```python
from build123d import *
from build123d.topology import SkipClean

# Parameters (mm, degrees)
CROQUIS1_R              = 15
CROQUIS1_R_2            = 11
SALIENTE_EXTRUIR1_DEPTH = 10
CROQUIS2_R              = 15
SALIENTE_EXTRUIR2_DEPTH = 1
CROQUIS3_R              = 15
CROQUIS3_R_2            = 12.25
SALIENTE_EXTRUIR3_DEPTH = 8.5


with BuildPart() as part:
    # Croquis1 → Saliente-Extruir1 (new body)
    with BuildSketch(Plane.XY):
        Circle(CROQUIS1_R)
        Circle(CROQUIS1_R_2, mode=Mode.SUBTRACT)
    extrude(amount=SALIENTE_EXTRUIR1_DEPTH)

    # Croquis2 → Saliente-Extruir2 (add, symmetric)
    with SkipClean():  # the faces are left unmerged after this step: merging them gives an invalid solid
        with BuildSketch(Plane(origin=(0, 0, 0), x_dir=(-1, 0, 0), z_dir=(0, 0, -1))):
            Circle(CROQUIS2_R)
        extrude(amount=SALIENTE_EXTRUIR2_DEPTH, both=True)

    # Croquis3 → Saliente-Extruir3 (add)
    with SkipClean():  # the faces are left unmerged after this step: merging them gives an invalid solid
        with BuildSketch(Plane.XY.offset(10)):
            with Locations(Location((0, 0, 0), (0, 0, 180))):
                Circle(CROQUIS3_R)
            Circle(CROQUIS3_R_2, mode=Mode.SUBTRACT)
        extrude(amount=SALIENTE_EXTRUIR3_DEPTH)


solid = part.part
```
CAD build for the part. Positions are in the model's coordinates, mm. A direction names the side the tool comes from. Coordinates: 2 decimals unless noted, no trailing zeros. Order: outer loops, then holes, each group sorted by start corner. A loop starts at its lowest first (then second) coordinate and runs counter-clockwise, first axis right, second up. Notation, with made-up numbers: (58, 13) - (82, 13) arc R17 ccw to (82, 21) - close; hole circle Ø2 at (25.25, 74). An arc over 180 degrees is marked (long way). Use a Markdown table: item, result. Add a question column.
(1) Saw through at B-B (x = -3.75). Give the cut face in (y, z).
(2) Flat gauge pins, fed straight in: pin 1 (6.5 mm diameter, centred on x = 1.5, y = 0.5, fed in from +Z); pin 2 (5 mm diameter, centred on y = -9.5, z = 11, fed in from +X); pin 3 (6 mm diameter, centred on x = 9, z = 9, fed in from -Y). Where does each tip first touch, or does it go through?
(3) Drill centre lines: line 1 along X through (y, z) = (0.25, 14); line 2 along Y through (x, z) = (0, 3.5). Where is each one in solid material? Low to high. Write a range as [from, to].
(4) Saw through at D-D (z = 11.75). Give the cut face in (x, y), then the cut area to 3 significant figures.
(5) Saw through at A-A (z = 6.5). Give the cut face in (x, y), then the cut area to 3 significant figures.
(6) Pull direction Y, two halves, no side cores. Call faces 3 (the face through (6, 11, 18.5)), 4 (the face through (-10, 5, 10)), 5 (the face through (0, 0, 1)): +Y half, -Y half, draft (parallel to the pull), parting line (faces both ways), or undercut.
(7) Which spindle directions (+Z, -Z, +X, -X, +Y, -Y) get a long thin tool onto all of the face, cutting with end or side? Do faces 1 (the face through (6.586, 10.329, 14.19)), 2 (the face through (0, 0, -1)). Say none if no direction does.
(8) Saw through at C-C (y = -4.25). Give the cut face in (x, z), then the cut area to 3 significant figures.
Solved:
| question | item | result |
|---|---|---|
| 1 | outline | (-14.52, -1) - (14.52, -1) - (14.52, 18.5) - (11.66, 18.5) - (11.66, 10) - (10.34, 10) - (10.34, 1) - (-10.34, 1) - (-10.34, 10) - (-11.66, 10) - (-11.66, 18.5) - (-14.52, 18.5) - close |
| 2 | pin 1 | stops at z = 1 |
| 2 | pin 2 | stops at x = 13.27 |
| 2 | pin 3 | stops at y = -13.75 |
| 3 | line 1 | x = [-15, -12.25], [12.25, 15] |
| 3 | line 2 | y = [-15, -11], [11, 15] |
| 4 | outline | circle Ø30 at (0, 0); hole circle Ø24.5 at (0, 0) |
| 4 | area | 235 mm² |
| 5 | outline | circle Ø30 at (0, 0); hole circle Ø22 at (0, 0) |
| 5 | area | 327 mm² |
| 6 | face 3 | draft |
| 6 | face 4 | undercut |
| 6 | face 5 | undercut |
| 7 | face 1 | +Z |
| 7 | face 2 | -Z, +X, -X, +Y, -Y |
| 8 | outline | (-14.39, -1) - (14.39, -1) - (14.39, 18.5) - (11.49, 18.5) - (11.49, 10) - (10.15, 10) - (10.15, 1) - (-10.15, 1) - (-10.15, 10) - (-11.49, 10) - (-11.49, 18.5) - (-14.39, 18.5) - close |
| 8 | area | 183 mm² |
